The model under review builds one solid part; all positions refer to its coordinate system, in mm. Face numbers are marked on the shaded views. A direction names the side the tool comes from. Coordinates: 2 decimals unless noted, no trailing zeros. Loops run counter-clockwise (first coordinate to the right, second up) from the corner with the lowest first, then second, coordinate; pieces in that order, holes last. Notation, with made-up numbers: (-33.5, 47.25) - (15.5, 47.25) arc R28 ccw to (15.5, 72.25) - close; hole circle Ø8 at (-7, 44.25). An arc over 180 degrees is marked (long way). Answer in a Markdown table with one row per item. Add a question column.
(1) Mouldability with a two-part tool opening along Y and no side actions: class the marked faces 4, 5, 6 and 7 as +Y half, -Y half, draft (parallel to the pull), parting line (faces both ways), or undercut.
(2) We need section B-B on y = 0. Write out the cut boundary in (x, z).
(3) For line 1 along X through (y, z) = (-8.25, 3.5); line 2 along Z through (x, y) = (-0.25, 0.5); line 3 along Y through (x, z) = (5.75, 2.5), list the stretches that pass through material, from the lowest coordinate up.
(4) For P1, Ø5, axis at x = 4.5, y = 0, coming from the -Z side; P2, Ø1, axis at x = -5, z = 1, coming from the -Y side; P3, Ø1.5, axis at y = 1.5, z = -1.5, coming from the +X side; P4, Ø1.2, axis at x = 5.5, z = -1, coming from the +Y side, all flat-tipped, find the tip position at first contact; note any pin that passes through.
(5) We need section C-C on z = -0.75. Write out the cut boundary in (x, y), plus the area to 3 significant figures.
(6) We need section D-D on x = -5. Write out the cut boundary in (y, z).
(7) We need section A-A on x = 5. Write out the cut boundary in (y, z).
(8) Machinability: for the marked faces 1, 2 and 3, which of the approach directions +Z, -Z, +X, -X, +Y, -Y give a long, thin tool a straight path to every point of the face, cutting with its end or side? Answer none if there is none.
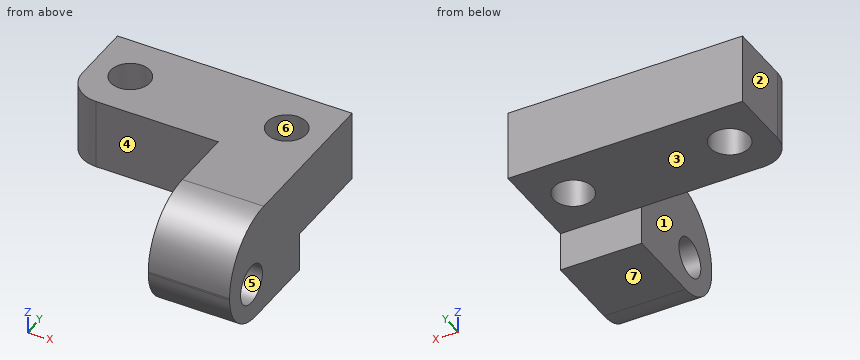
from build123d import *

# Parameters (mm, degrees)
SKETCH_1_W         = 15
SKETCH_1_H         = 6
EXTRUDE_1_DEPTH    = 4.5
HOLE_WIZARD_M3_1_D = 2.5
EXTRUDE_START      = 2.3
SKETCH_5_W         = 7
SKETCH_5_H         = 8
EXTRUDE_2_DEPTH    = 5.2
FILLET_1_R         = 3.9
FILLET_2_R         = 3
HOLE_WIZARD_M3_2_D = 2.5
FILLET_3_R         = 2


with BuildPart() as part:
    # 草图1 → 凸台-拉伸1 (new body)
    with BuildSketch(Plane.XY):
        Rectangle(SKETCH_1_W, SKETCH_1_H)
    extrude(amount=EXTRUDE_1_DEPTH)

    # M3 螺纹孔1 (through all)
    with Locations(Plane.XY.offset(4.5)):
        with Locations((-5, 0), (5, 0)):
            Hole(HOLE_WIZARD_M3_1_D / 2)

    # 草图5 → 凸台-拉伸2 (add)
    with BuildSketch(Plane(origin=(0, 0, 0), x_dir=(0, 0, -1), z_dir=(1, 0, 0)).offset(EXTRUDE_START)):
        with Locations((-1, -7)):
            Rectangle(SKETCH_5_W, SKETCH_5_H)
    extrude(amount=EXTRUDE_2_DEPTH)

    # 圆角1
    fillet_1_edges = [part.edges().sort_by_distance(p)[0] for p in [
        (4.9, -11, 4.5),
    ]]
    fillet(fillet_1_edges, radius=FILLET_1_R)

    # 圆角2
    fillet_2_edges = [part.edges().sort_by_distance(p)[0] for p in [
        (4.9, -11, -2.5),
    ]]
    fillet(fillet_2_edges, radius=FILLET_2_R)

    # M3 螺纹孔2 (through all)
    with Locations(Plane.ZY.offset(-2.3)):
        with Locations((0, -8.5)):
            Hole(HOLE_WIZARD_M3_2_D / 2)

    # 圆角3
    fillet_3_edges = [part.edges().sort_by_distance(p)[0] for p in [
        (-7.5, -3, 2.25),
    ]]
    fillet(fillet_3_edges, radius=FILLET_3_R)


solid = part.part
Outcome:
| question | item | result |
|---|---|---|
| 1 | face 4 | -Y half |
| 1 | face 5 | undercut |
| 1 | face 6 | undercut |
| 1 | face 7 | draft |
| 2 | outline | (-7.5, 0) - (-6.25, 0) - (-6.25, 4.5) - (-7.5, 4.5) - close; (-3.75, 0) - (3.75, 0) - (3.75, 4.5) - (-3.75, 4.5) - close; (6.25, 0) - (7.5, 0) - (7.5, 4.5) - (6.25, 4.5) - close |
| 3 | line 1 | 2.3 to 7.5 |
| 3 | line 2 | 0 to 4.5 |
| 3 | line 3 | -10.51 to -1, 1 to 3 |
| 4 | P1 | z = 0 |
| 4 | P2 | y = -3 |
| 4 | P3 | through |
| 4 | P4 | y = -3 |
| 5 | outline | (2.3, -10.73) - (7.5, -10.73) - (7.5, -9.5) - (2.3, -9.5) - close; (2.3, -7.5) - (7.5, -7.5) - (7.5, -3) - (2.3, -3) - close |
| 5 | area | 29.8 mm² |
| 6 | outline | (-3, 0) - (-1.25, 0) - (-1.25, 4.5) - (-3, 4.5) - close; (1.25, 0) - (3, 0) - (3, 4.5) - (1.25, 4.5) - close |
| 7 | outline | (-11, 0.5) arc R3 ccw to (-8, -2.5) - (-3, -2.5) - (-3, 0) - (-1.25, 0) - (-1.25, 4.5) - (-7.1, 4.5) arc R3.9 ccw to (-11, 0.6) - close; (1.25, 0) - (3, 0) - (3, 4.5) - (1.25, 4.5) - close; hole circle Ø2.5 at (-8.5, 0) |
| 8 | face 1 | +Z, -Z, -X, -Y |
| 8 | face 2 | +Z, -Z, -X, +Y, -Y |
| 8 | face 3 | -Z, +X, -X, +Y |
